Input: dimensioned drawing with shaded views. Units: mm. Origin: part minimum x, y, z. A direction names the side the tool comes from. Give positions to 0.01 mm unless a question says otherwise; leave off trailing zeros. Write each loop counter-clockwise with the first axis right and the second up, starting at its lowest first coordinate (ties: lowest second). Pieces come first, ordered by that corner, then holes. Notation, with made-up numbers: (-11.75, -40) -> (7.25, -40) arc R32 cw to (7.25, -1) -> close; hole circle Ø1 at (-28, -18.75). An arc over 180 degrees is marked (long way). Answer in a Markdown table with one row per item. Add a question column.
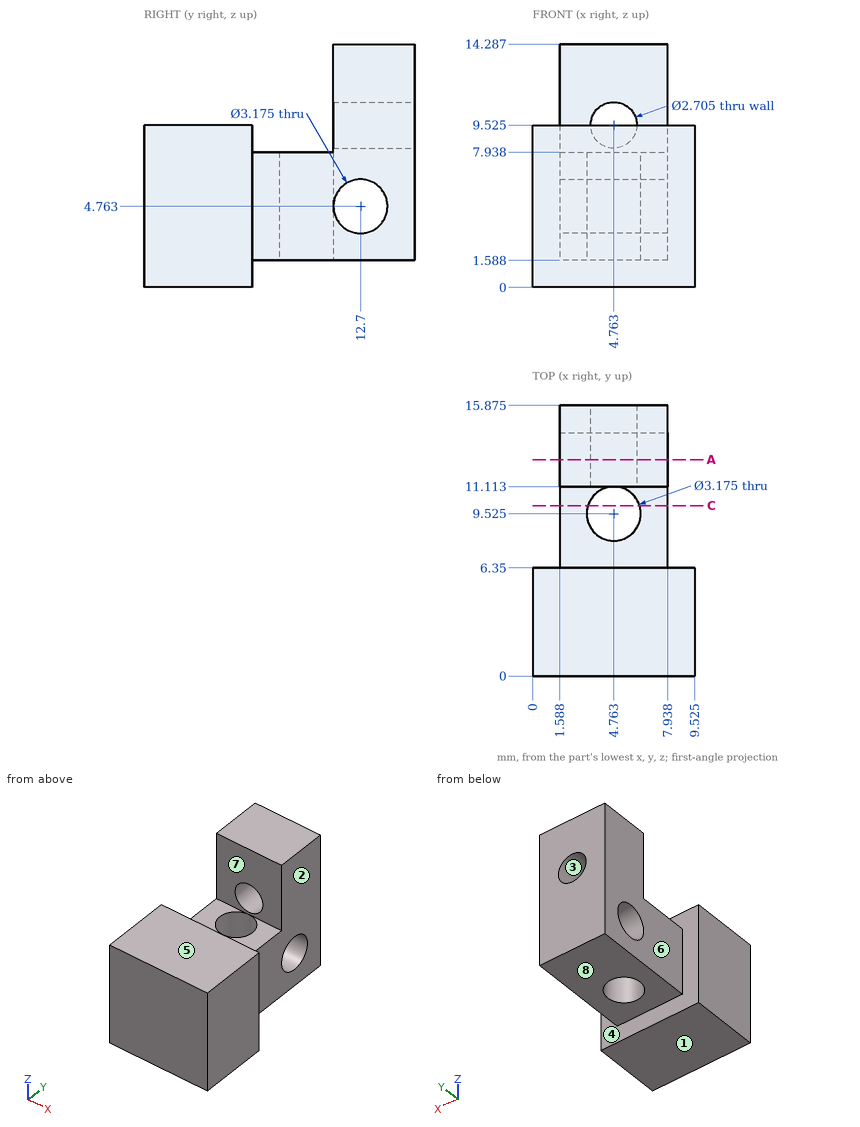
Q1. Section C-C on y = 10. Return loops of the section in (x, z), and give its area (3 significant figures).
Q2. Section A-A on y = 12.7. Count the separate pieces of the cut face and the enclosed holes in it.
Q3. Access query for the marked faces 4, 5, 6, 7 and 8. Directions: +Z, -Z, +X, -X, +Y, -Y. A direction counts if a zero-diameter tool reaches every point of the face in a straight line with its end or side. Return the directions, or none.
Q4. Pull-direction query (X, two-part tool) for the marked faces 1, 2 and 3; classes: +X half, -X half, draft (parallel to the pull), parting line (faces both ways), or undercut.
Q5. Contact query for flat-ended pins moving along their axis: pin 1 Ø2 at (x, z) = (4.76, 9.52) entering from +Y; pin 2 Ø3 at (y, z) = (12.7, 4.76) entering from -X; pin 3 Ø1.5 at (x, y) = (7.5, 9.5) entering from +Z; pin 4 Ø1.9 at (x, y) = (6, 12.5) entering from -Z. Output: stop coordinate, or through.
Q6. Line query: probe 1 along Z at (x, y) = (4, 2.75) (1 decimal); probe 2 along X at (y, z) = (7.5, 5); probe 3 along Y at (x, z) = (7.5, 1.25). Output: solid intervals per line, ascending. Write a range as from..to.
Checks:
| question | item | result |
|---|---|---|
| 1 | outline | (1.59, 1.59) -> (3.25, 1.59) -> (3.25, 7.94) -> (1.59, 7.94) -> close; (6.28, 1.59) -> (7.94, 1.59) -> (7.94, 7.94) -> (6.28, 7.94) -> close |
| 1 | area | 21.1 mm^2 |
| 2 | separate pieces | 2 |
| 2 | enclosed holes | 1 |
| 3 | face 4 | none |
| 3 | face 5 | +Z, +X, -X, -Y |
| 3 | face 6 | +Z, -Z, -X, +Y |
| 3 | face 7 | +Z, +X, -X |
| 3 | face 8 | -Z, +X, -X, +Y |
| 4 | face 1 | draft |
| 4 | face 2 | +X half |
| 4 | face 3 | undercut |
| 5 | pin 1 | y = 6.35 |
| 5 | pin 2 | through |
| 5 | pin 3 | z = 7.94 |
| 5 | pin 4 | z = 1.59 |
| 6 | probe 1 | 0..9.5 |
| 6 | probe 2 | 1.59..7.94 |
| 6 | probe 3 | 0..6.35 |
